Here's how the part is built. I have some questions about the finished solid (model axes, mm). Face numbers are marked on the shaded views. A direction names the side the tool comes from. Round coordinates to 2 decimals unless told otherwise and drop trailing zeros. Write each loop counter-clockwise with the first axis right and the second up, starting at its lowest first coordinate (ties: lowest second). Pieces come first, ordered by that corner, then holes. Notation, with made-up numbers: (-9.5, -17) -> (41.5, -17) arc R29 ccw to (41.5, 9) -> close; hole circle Ø9 at (-18, 62). An arc over 180 degrees is marked (long way). Answer in a Markdown table with one row per item.
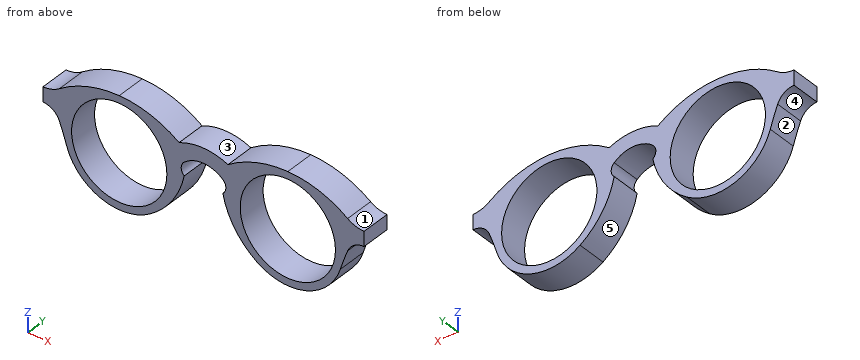
from build123d import *

# Parameters (mm, degrees)
F0_R     = 20.6375
F1_DEPTH = 12.7


with BuildPart() as f1:
    # F0 (on Front) → F1 (new body)
    with BuildSketch(Plane.XZ):
        with BuildLine():
            ThreePointArc((0, 23.8125), (16.83798, 16.83798), (23.8125, 0))
            ThreePointArc((23.8125, 0), (21.037854, -11.155441), (13.360522, -19.711205))
            ThreePointArc((13.360522, -19.711205), (22.941831, -10.040538), (28.143111, 2.54))
            ThreePointArc((28.143111, 2.54), (26.841467, 5.411069), (28.143111, 8.282137))
            ThreePointArc((28.143111, 8.282137), (36.5125, 11.43), (44.881889, 8.282137))
            ThreePointArc((44.881889, 8.282137), (46.183533, 5.411069), (44.881889, 2.54))
            ThreePointArc((44.881889, 2.54), (50.083169, -10.040538), (59.664478, -19.711205))
            ThreePointArc((59.664478, -19.711205), (50.260903, 6.987921), (73.025, 23.8125))
            ThreePointArc((73.025, 23.8125), (59.407251, 21.675139), (47.099111, 15.468605))
            ThreePointArc((47.099111, 15.468605), (36.5125, 17.78), (25.925889, 15.468605))
            ThreePointArc((25.925889, 15.468605), (13.617749, 21.675139), (0, 23.8125))
        make_face()
        with BuildLine():
            ThreePointArc((13.360522, -19.711205), (21.037854, -11.155441), (23.8125, 0))
            ThreePointArc((23.8125, 0), (16.83798, 16.83798), (0, 23.8125))
            ThreePointArc((0, 23.8125), (-19.180682, 14.111577), (-22.73341, -7.087116))
            ThreePointArc((-22.73341, -7.087116), (-7.861594, -22.477333), (13.360522, -19.711205))
        make_face()
        Circle(F0_R, mode=Mode.SUBTRACT)
        with BuildLine():
            ThreePointArc((-22.73341, -7.087116), (-19.180682, 14.111577), (0, 23.8125))
            ThreePointArc((0, 23.8125), (-13.617749, 21.675139), (-25.925889, 15.468605))
            ThreePointArc((-25.925889, 15.468605), (-29.29377, 13.770308), (-33.02, 13.185461))
            Line((-33.02, 13.185461), (-33.02, 6.835461))
            ThreePointArc((-33.02, 6.835461), (-28.726536, 5.510743), (-25.925889, 1.997185))
            ThreePointArc((-25.925889, 1.997185), (-24.248459, -2.516433), (-22.73341, -7.087116))
        make_face()
        with BuildLine():
            ThreePointArc((96.8375, 0), (89.86298, 16.83798), (73.025, 23.8125))
            ThreePointArc((73.025, 23.8125), (50.260903, 6.987921), (59.664478, -19.711205))
            ThreePointArc((59.664478, -19.711205), (80.886594, -22.477333), (95.75841, -7.087116))
            ThreePointArc((95.75841, -7.087116), (96.566182, -3.584399), (96.8375, 0))
        make_face()
        with Locations((73.025, 0)):
            Circle(F0_R, mode=Mode.SUBTRACT)
        with BuildLine():
            ThreePointArc((98.950889, 15.468605), (86.642749, 21.675139), (73.025, 23.8125))
            ThreePointArc((73.025, 23.8125), (89.86298, 16.83798), (96.8375, 0))
            ThreePointArc((96.8375, 0), (96.566182, -3.584399), (95.75841, -7.087116))
            ThreePointArc((95.75841, -7.087116), (97.273459, -2.516433), (98.950889, 1.997185))
            ThreePointArc((98.950889, 1.997185), (101.751536, 5.510743), (106.045, 6.835461))
            Line((106.045, 6.835461), (106.045, 13.185461))
            ThreePointArc((106.045, 13.185461), (102.31877, 13.770308), (98.950889, 15.468605))
        make_face()
    extrude(amount=F1_DEPTH)


solid = f1.part
1) I want a section at C-C, the plane z = 0. List the corners of the cut face in (x, y) for me, and give its area (3 significant figures).
Response:
| item | result |
|---|---|
| outline | (-25.16, -12.7) -> (-20.64, -12.7) -> (-20.64, 0) -> (-25.16, 0) -> close; (20.64, -12.7) -> (27.54, -12.7) -> (27.54, 0) -> (20.64, 0) -> close; (45.49, -12.7) -> (52.39, -12.7) -> (52.39, 0) -> (45.49, 0) -> close; (93.66, -12.7) -> (98.19, -12.7) -> (98.19, 0) -> (93.66, 0) -> close |
| area | 290 mm^2 |
2) I want a section at A-A, the plane y = -9.25. Count the separate pieces of the cut face and the enclosed holes in it, and give its area (3 significant figures).
Response:
| item | result |
|---|---|
| separate pieces | 1 |
| enclosed holes | 2 |
| area | 1,660 mm^2 |
3) I need wall thicknesses on line 1 (X direction, y = -9.25, z = 9) (3 decimals); line 2 (X direction, y = -7, z = -9); line 3 (Z direction, x = 4, y = -12). Which ranges of each line are inside material? Lowest first, please. Write a range as [from, to].
Response:
| item | result |
|---|---|
| line 1 | x = [-33.02, -18.572], [18.572, 29.041], [43.984, 54.453], [91.597, 106.045] |
| line 2 | x = [-22.05, -18.57], [18.57, 23.61], [49.42, 54.45], [91.6, 95.07] |
| line 3 | z = [-23.47, -20.25], [20.25, 23.63] |
4) Which directions (+Z, -Z, +X, -X, +Y, -Y) give clear straight access to the entire face, cutting with the end or side of a thin tool? Please do the marked faces 4 and 5.
Response:
| item | result |
|---|---|
| face 4 | -Z, -X, +Y, -Y |
| face 5 | -Z, +Y, -Y |
5) We'd pull the mould along X, two halves only. Please class the marked faces 1, 2 and 3: +X half, -X half, draft (parallel to the pull), parting line (faces both ways), or undercut.
Response:
| item | result |
|---|---|
| face 1 | +X half |
| face 2 | -X half |
| face 3 | undercut |
6) I want a section at B-B, the plane x = 15. List the corners of the cut face in (y, z) for me.
Response:
| item | result |
|---|---|
| outline | (-12.7, -18.53) -> (0, -18.53) -> (0, -14.17) -> (-12.7, -14.17) -> close; (-12.7, 14.17) -> (0, 14.17) -> (0, 21.21) -> (-12.7, 21.21) -> close |
7) I want a section at D-D, the plane z = -17. List the corners of the cut face in (x, y) for me.
Response:
| item | result |
|---|---|
| outline | (-16.67, -12.7) -> (-11.7, -12.7) -> (-11.7, 0) -> (-16.67, 0) -> close; (11.7, -12.7) -> (16.86, -12.7) -> (16.86, 0) -> (11.7, 0) -> close; (56.16, -12.7) -> (61.32, -12.7) -> (61.32, 0) -> (56.16, 0) -> close; (84.73, -12.7) -> (89.7, -12.7) -> (89.7, 0) -> (84.73, 0) -> close |
8) For pin 1 (3 mm diameter, centred on x = 18.5, z = 0.5, fed in from +Y); pin 2 (1 mm diameter, centred on x = 26, y = -2, fed in from -Z); pin 3 (2 mm diameter, centred on x = 32, y = -11, fed in from +Z); pin 4 (1.5 mm diameter, centred on x = 54, y = -7, fed in from -Z), each with a flat end and sliding along its axis, tell me the tip position at first contact or that it passes through.
Response:
| item | result |
|---|---|
| pin 1 | passes through |
| pin 2 | stops at z = -5.49 |
| pin 3 | stops at z = 17.54 |
| pin 4 | stops at z = -15.69 |
